from build123d import *

# Parameters (mm, degrees)
SKETCH_1_W          = 32
SKETCH_1_H          = 10
SKETCH_1_R          = 2.395
EXTRUDE_2_DEPTH     = 6.36
FILLET_4_R          = 5
EXTRUDE_3_DEPTH     = 6.36
FILLET_5_R          = 8
FILLET_6_R          = 8
SKETCH_3_R          = 130
CUT_EXTRUDE_2_DEPTH = 6.36


with BuildPart() as part:
    # 草图1 → 凸台-拉伸2 (new body)
    with BuildSketch(Plane(origin=(0, 0, 0), x_dir=(1, 0, 0), z_dir=(0, 1, 0))):
        Rectangle(SKETCH_1_W, SKETCH_1_H)
        with Locations(Location((11, 0, 0), (0, 0, 90))):
            Circle(SKETCH_1_R, mode=Mode.SUBTRACT)
        with Locations(Location((-11, 0, 0), (0, 0, 90))):
            Circle(SKETCH_1_R, mode=Mode.SUBTRACT)
    extrude(amount=EXTRUDE_2_DEPTH)

    # 圆角4
    fillet_4_edges = [part.edges().sort_by_distance(p)[0] for p in [
        (-16, 3.18, 5),
        (-16, 3.18, -5),
    ]]
    fillet(fillet_4_edges, radius=FILLET_4_R - 0.0001)  # a hair under: the kernel refuses the full size

    # 草图2 → 凸台-拉伸3 (add)
    with BuildSketch(Plane(origin=(0, 0, 0), x_dir=(1, 0, 0), z_dir=(0, 1, 0))):
        Polygon((11, 5), (98.421265934, 26.389770044), (123.676298315, 22.569036945), (123.676298315, 14.569036945), (115.905519121, 12.667724053), (18.770779194, -11.098687107), (11, -13), (11, -5), (16, 0), align=None)
    extrude(amount=EXTRUDE_3_DEPTH)

    # 圆角5
    fillet_5_edges = [part.edges().sort_by_distance(p)[0] for p in [
        (123.676298315, 3.18, -22.569036945),
        (11, 3.18, 5),
    ]]
    fillet(fillet_5_edges, radius=FILLET_5_R - 0.0001)  # a hair under: the kernel refuses the full size

    # 圆角6
    fillet_6_edges = [part.edges().sort_by_distance(p)[0] for p in [
        (11, 3.18, -5),
        (98.421265934, 3.18, -26.389770044),
    ]]
    fillet(fillet_6_edges, radius=FILLET_6_R)

    # 草图3 → 切除-拉伸2 (cut)
    with BuildSketch(Plane(origin=(0, 0, 0), x_dir=(1, 0, 0), z_dir=(0, 1, 0))):
        with Locations((95.857842549, -115.777169439)):
            Circle(SKETCH_3_R)
    extrude(amount=CUT_EXTRUDE_2_DEPTH, mode=Mode.SUBTRACT)


solid = part.part
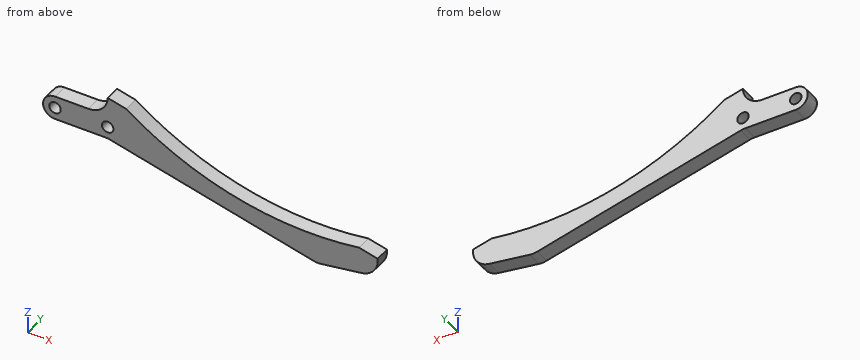
The listing builds one solid part. Answer for the finished solid, in the listing's coordinates (mm). Coordinates: 2 decimals unless noted, no trailing zeros. Write each loop counter-clockwise with the first axis right and the second up, starting at its lowest first coordinate (ties: lowest second). Pieces come first, ordered by that corner, then holes. Notation, with made-up numbers: (36.25, 76) - (42.25, 76) arc R9 ccw to (42.25, 93) - close; hole circle Ø6 at (-24, 48). An arc over 180 degrees is marked (long way). Put each result on its own line as item: value.
1. The part is cut by section C-C on z = -21. Give the vertices of the cut face in (x, y).
Answer sheet:
outline: (76.39, 0) - (121.66, 0) - (121.66, 6.36) - (76.39, 6.36) - close
2. Find the intervals of material crossed by line 1 along X through (y, z) = (3.25, 0) (3 decimals); line 2 along Z through (x, y) = (-11, 3.75) (3 decimals); line 3 along Z through (x, y) = (-5.5, 2), in increasing order. Write a range as from..to.
Answer sheet:
line 1: x = -16..-13.395, -8.605..8.605, 13.395..36.734
line 2: z = -5..-2.395, 2.395..5
line 3: z = -5..5
3. Flat-ended cylindrical pins translate along their axes: pin 1 Ø1.5 at (y, z) = (4, 1) entering from +X; pin 2 Ø2 at (x, y) = (102, 1) entering from -Z; pin 3 Ø1 at (y, z) = (2.5, 3.5) entering from -X. Find the tip coordinate at first contact, or state that the pin passes through.
Answer sheet:
pin 1: stops at x = 36.25
pin 2: stops at z = -26
pin 3: stops at x = -15
4. The part is cut by section A-A on y = 5. State how many separate pieces and enclosed holes the cut face has, plus the area to 3 significant figures.
Answer sheet:
separate pieces: 1
enclosed holes: 2
area: 1,460 mm^2
5. The part is cut by section B-B on x = -1. Give the vertices of the cut face in (y, z), plus the area to 3 significant figures.
Answer sheet:
outline: (0, -5) - (6.36, -5) - (6.36, 5) - (0, 5) - close
area: 63.6 mm^2
